Here's how the part is built. I have some questions about the finished solid (model axes, mm). A direction names the side the tool comes from. Coordinates: 2 decimals unless noted, no trailing zeros. Loops run counter-clockwise (first coordinate to the right, second up) from the corner with the lowest first, then second, coordinate; pieces in that order, holes last.
Autodesk Inventor part; units mm, degrees
ref_plane "YZ Plane" through (0, 0, 0) normal (1, 0, 0) x (0, 1, 0)
ref_plane "XZ Plane" through (0, 0, 0) normal (0, 1, 0) x (-1, 0, 0)
ref_plane "XY Plane" through (0, 0, 0) normal (0, 0, 1) x (1, 0, 0)
sketch "Sketch1" plane through (0, 0, 0) normal (0, 1, 0) x (-1, 0, 0)
  line L0 (0, 0) -> (-35, 0)
  line L1 (-35, 0) -> (-35, -5)
  line L2 (-5, -35) -> (0, -35)
  line L3 (0, -35) -> (0, 0)
  line L4 (-5, -5) -> (-35, -5)
  line L5 (-5, -35) -> (-5, -5)
  line L6 (-35, -5) -> (-5, -35)
  point P0 (-15, -15)
  dimension "d2" = 5
  dimension "d3" = 5
  dimension "d4" = 10
  dimension "d5" = 10
  dimension "d6" = 35
  dimension "d7" = 35
extrude "Extrusion1" add sketch "Sketch1" along normal blind 20 contours L3 L2 L5 L4 L1 L0
extrude "Extrusion2" add sketch "Sketch1" along normal blind 5 contours L4 L5 L6
sketch "Sketch2" plane through (5, 20, -5) normal (1, 0, 0) x (0, 0, -1)
  point P0 (-5, -20)
ref_plane "Work Plane1" through (5, 20, -5) normal (0.7071, 0, 0.7071) x (0, -1, 0)
sketch "Sketch3" plane through (5, 20, -5) normal (1, 0, 0) x (0, 0, -1)
  line L0 (0, 0) -> (30, 0)
  line L1 (0, -15) -> (0, 0)
  line L2 (30, -15) -> (30, 0)
  point P0 (-5, -20)
  point P1 (7, -10)
  point P2 (23, -10)
  dimension "d12" = 10
  dimension "d13" = 7
  dimension "d14" = 7
  dimension "d15" = 10
sketch "Sketch4" plane through (0, 5, 0) normal (0, 1, 0) x (1, 0, 0)
  point P0 (0, 0)
  point P1 (15, 15)
hole "Hole1" at (15, 5, -15) direction (0, -1, 0) diameter 4.5 end through all counterbore diameter 8 counterbore depth 2
hole "Hole2" at (5, 10, -12) at (5, 10, -28) direction (-1, 0, 0) diameter 4.5 end through all counterbore diameter 8 counterbore depth 2
mirror "Mirror1" about plane through (5, 20, -5) normal (0.7071, 0, 0.7071) of "Hole2"
properties part number "angle_90_profile_2020"
1. On a 3-axis mill with a long thin cutter (end or side, diameter ignored), from which of +Z, -Z, +X, -X, +Y, -Y can I reach the whole of each face in a straight line? I mean faces 1 (the flat face through (17, 10, 0)), 2 (the flat face through (17, 3, -13)), 3 (the flat face through (5, 12, -20)), 4 (the flat face through (3, 12, -14)), 5 (the cylindrical face through (24, 10, -4)). Say none if no direction works.
2. I want a section at C-C (x = 4.5). Please give me the cut outline in (y, z).
3. I need wall thicknesses on line 1 along X through (y, z) = (10, -3.45); line 2 along Y through (x, z) = (3.95, -28); line 3 along X through (y, z) = (10, -0.9). Which ranges of each line are inside material? Lowest first, please.
4. I want a section at A-A (x = 28). Please give me the cut outline in (y, z), then the cut area to 4 significant figures.
5. I want a section at B-B (z = -28). Please give me the cut outline in (x, y).
6. For pin 1 (4 mm diameter, centred on x = 13.5, y = 9, fed in from -Z); pin 2 (5 mm diameter, centred on y = 10, z = -28, fed in from +X); pin 3 (12 mm diameter, centred on x = 25.5, z = -27.5, fed in from -Y); pin 4 (2 mm diameter, centred on y = 5.5, z = -10, fed in from +X), each with a flat end and sliding along its axis, tell me the tip position at first contact or that it passes through.
7. I want a section at D-D (y = 10). Give the number of separate pieces and of enclosed holes in the cut face, then the cut area to 3 significant figures.
8. We'd pull the mould along Z, two halves only. Please class faces 6 (the flat face through (10, 12, -3)), 7 (the flat face through (0, 10, -18)), 8 (the flat face through (3, 12, -30)): +Z half, -Z half, draft (parallel to the pull), parting line (faces both ways), or undercut.
Response values:
1. face 1: +Z, +X, -X, +Y, -Y
1. face 2: +Y
1. face 3: -Z, +X, +Y
1. face 4: +X
1. face 5: -Z
2. outline: (0, -35) - (20, -35) - (20, 0) - (0, 0) - close; hole circle Ø8 at (10, -28); hole circle Ø8 at (10, -12)
3. line 1: x = 0 to 8, 16 to 24, 32 to 35
3. line 2: y = 0 to 6, 14 to 20
3. line 3: x = 0 to 9.75, 14.25 to 25.75, 30.25 to 35
4. outline: (0, -12) - (5, -12) - (5, -5) - (6, -5) - (6, -3) - (7.75, -3) - (7.75, 0) - (0, 0) - close; (12.25, -3) - (14, -3) - (14, -5) - (20, -5) - (20, 0) - (12.25, 0) - close
4. area: 105.5 mm2
5. outline: (0, 0) - (12, 0) - (12, 5) - (5, 5) - (5, 6) - (3, 6) - (3, 7.75) - (0, 7.75) - close; (0, 12.25) - (3, 12.25) - (3, 14) - (5, 14) - (5, 20) - (0, 20) - close
6. pin 1: stops at z = -3
6. pin 2: stops at x = 3
6. pin 3: passes through
6. pin 4: stops at x = 30.87
7. separate pieces: 5
7. enclosed holes: 0
7. area: 207 mm2
8. face 6: -Z half
8. face 7: draft
8. face 8: undercut
